Here's how the part is built. I have some questions about the finished solid (model axes, mm). Face numbers are marked on the shaded views. A direction names the side the tool comes from. Give positions to 0.01 mm unless a question says otherwise; leave off trailing zeros. Order: outer loops, then holes, each group sorted by start corner. A loop starts at its lowest first (then second) coordinate and runs counter-clockwise, first axis right, second up. Notation, with made-up numbers: (70.5, 73) - (78.5, 73) arc R31 cw to (78.5, 107) - close; hole circle Ø7 at (25, -8). An arc over 180 degrees is marked (long way). One line per question, with ' | ' between items.
from build123d import *

# Parameters (mm, degrees)
EXTRUDE_1_DEPTH              = 35
CUT_EXTRUDE_2_DEPTH          = 30
SKETCH_2_R                   = 10
SKETCH_2_R_2                 = 15
CUT_EXTRUDE_1_DEPTH          = 1
CUT_EXTRUDE_1_DEPTH_BACK     = 36
EXTRUDE_2_DEPTH              = 5
CUT_EXTRUDE_4_REACH          = 42
SKETCH_11_R                  = 6
EXTRUDE_4_DEPTH              = 35
FILLET_1_R                   = 10
HOLE_WIZARD_M3_1_D           = 2.5
HOLE_WIZARD_M2_1_D           = 1.6
HOLE_WIZARD_M4_1_D           = 3.3
HOLE_WIZARD_M4_2_D           = 4.5
HOLE_WIZARD_M4_2_DEPTH       = 40
HOLE_WIZARD_M4_2_CBORE_D     = 9
HOLE_WIZARD_M4_2_CBORE_DEPTH = 33.1
HOLE_WIZARD_M4_2_TIP         = 1.351936393


with BuildPart() as part:
    # 스케치1 → 보스-돌출1 (new body)
    with BuildSketch(Plane(origin=(0, 0, 0), x_dir=(0, 0, -1), z_dir=(1, 0, 0))):
        with BuildLine():
            Line((-48.263014716, 12.710470067), (81.736985284, 12.710470067))
            ThreePointArc((81.736985284, 12.710470067), (116.736985284, -22.289529933), (81.736985284, -57.289529933))
            Line((81.736985284, -57.289529933), (-48.263014716, -57.289529933))
            ThreePointArc((-48.263014716, -57.289529933), (-83.263014716, -22.289529933), (-48.263014716, 12.710470067))
        make_face()
    extrude(amount=-EXTRUDE_1_DEPTH)

    # 스케치3 → 컷-돌출2 (cut)
    with BuildSketch(Plane.ZY.offset(35)):
        with BuildLine():
            Line((48.263014716, 7.710470067), (-81.736985284, 7.710470067))
            ThreePointArc((-81.736985284, 7.710470067), (-111.736985284, -22.289529933), (-81.736985284, -52.289529933))
            Line((-81.736985284, -52.289529933), (48.263014716, -52.289529933))
            ThreePointArc((48.263014716, -52.289529933), (78.263014716, -22.289529933), (48.263014716, 7.710470067))
        make_face()
    extrude(amount=-CUT_EXTRUDE_2_DEPTH, mode=Mode.SUBTRACT)

    # 스케치2 → 컷-돌출1 (cut, two sides)
    with BuildSketch(Plane(origin=(0, 0, 0), x_dir=(0, 0, -1), z_dir=(1, 0, 0))) as cut_extrude_1_sk:
        with Locations((-23.263014716, -22.302890454)):
            Circle(SKETCH_2_R)
        with Locations((81.736985284, -22.302890454)):
            Circle(SKETCH_2_R_2)
    extrude(amount=CUT_EXTRUDE_1_DEPTH, mode=Mode.SUBTRACT)
    extrude(cut_extrude_1_sk.sketch, amount=-CUT_EXTRUDE_1_DEPTH_BACK, mode=Mode.SUBTRACT)

    # 스케치6 → 보스-돌출2 (add)
    with BuildSketch(Plane.ZY.offset(35)):
        with BuildLine():
            Line((-81.736985284, -54.289529933), (48.263014716, -54.289529933))
            ThreePointArc((48.263014716, -54.289529933), (80.263014716, -22.289529933), (48.263014716, 9.710470067))
            Line((48.263014716, 9.710470067), (-81.736985284, 9.710470067))
            ThreePointArc((-81.736985284, 9.710470067), (-113.736985284, -22.289529933), (-81.736985284, -54.289529933))
        make_face()
        with BuildLine():
            Line((-81.736985284, -52.289529933), (48.263014716, -52.289529933))
            ThreePointArc((48.263014716, -52.289529933), (78.263014716, -22.289529933), (48.263014716, 7.710470067))
            Line((48.263014716, 7.710470067), (-81.736985284, 7.710470067))
            ThreePointArc((-81.736985284, 7.710470067), (-111.736985284, -22.289529933), (-81.736985284, -52.289529933))
        make_face(mode=Mode.SUBTRACT)
    extrude(amount=EXTRUDE_2_DEPTH)

    # 스케치8 → 컷-돌출4 (cut, up to next)
    with BuildSketch(Plane(origin=(0, 0, 0), x_dir=(0, 0, -1), z_dir=(1, 0, 0)), mode=Mode.PRIVATE) as cut_extrude_4_sk1:
        with BuildLine():
            ThreePointArc((76.560604382, -41.608046459), (97.60405209, -10.114301353), (61.736985284, -22.289529933))
            ThreePointArc((61.736985284, -22.289529933), (59.236985284, -24.789529933), (56.736985284, -22.289529933))
            ThreePointArc((56.736985284, -22.289529933), (101.570818791, -7.070494208), (75.266509157, -46.43767559))
            ThreePointArc((75.266509157, -46.43767559), (73.498742204, -43.375813412), (76.560604382, -41.608046459))
        make_face()
    cut_extrude_4_tool1 = extrude(cut_extrude_4_sk1.sketch, amount=-CUT_EXTRUDE_4_REACH, mode=Mode.PRIVATE) & part.part
    add(cut_extrude_4_tool1.solids().sort_by_distance((0, -43.558826, -74.181755))[0], mode=Mode.SUBTRACT)

    # 스케치11 → 보스-돌출4 (add)
    with BuildSketch(Plane.ZY.offset(5)):
        with Locations((-16.736985284, -47.289529933)):
            Circle(SKETCH_11_R)
        with Locations((-16.736985284, 2.710470067)):
            Circle(SKETCH_11_R)
    extrude(amount=EXTRUDE_4_DEPTH)

    # 필렛1
    fillet_1_edges = [part.edges().sort_by_distance(p)[0] for p in [
        (-22.5, -52.289529933, -20.053610075),
        (-22.5, -52.289529933, -13.420360494),
        (-22.5, 7.710470067, -13.420360494),
        (-22.5, 7.710470067, -20.053610075),
    ]]
    fillet(fillet_1_edges, radius=FILLET_1_R)

    # M3 나사 구멍1 (through all)
    with Locations(Plane.ZY.offset(5)):
        with Locations((-62.442692702, -31.965687796), (-68.870568799, -39.626132227)):
            Hole(HOLE_WIZARD_M3_1_D / 2)

    # M2 나사 구멍1 (through all)
    with Locations(Plane.ZY.offset(5)):
        with Locations((-95.142763039, -11.054107284)):
            Hole(HOLE_WIZARD_M2_1_D / 2)

    # M4 나사 구멍1 (through all)
    with Locations(Plane(origin=(0, 0, 0), x_dir=(0, 0, -1), z_dir=(1, 0, 0))):
        with Locations((-53.263014716, -7.302890454), (-53.263014716, -22.302890454), (-53.263014716, -37.302890454), (-33.869616434, -32.909492171), (-33.869616434, -11.696288736), (-12.656412998, -11.696288736), (-12.656412998, -32.909492171)):
            Hole(HOLE_WIZARD_M4_1_D / 2)

    # M4 남비 머리 나사용 카운터보어2
    with Locations(Plane(origin=(0, 0, 0), x_dir=(0, 0, -1), z_dir=(1, 0, 0))):
        with Locations((16.736985284, 2.710470067), (16.736985284, -47.289529933)):
            CounterBoreHole(HOLE_WIZARD_M4_2_D / 2, HOLE_WIZARD_M4_2_CBORE_D / 2, HOLE_WIZARD_M4_2_CBORE_DEPTH, depth=HOLE_WIZARD_M4_2_DEPTH)
            with Locations((0, 0, -(HOLE_WIZARD_M4_2_DEPTH + HOLE_WIZARD_M4_2_TIP / 2))):  # 118° drill point
                Cone(0, HOLE_WIZARD_M4_2_D / 2, HOLE_WIZARD_M4_2_TIP, mode=Mode.SUBTRACT)


solid = part.part
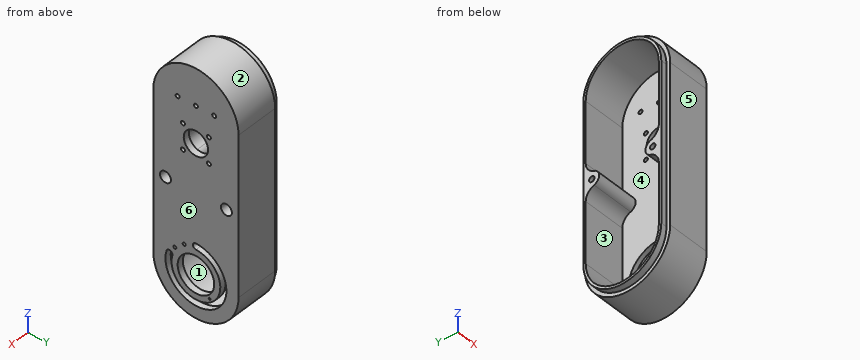
1) On a 3-axis mill with a long thin cutter (end or side, diameter ignored), from which of +Z, -Z, +X, -X, +Y, -Y can I reach the whole of each face in a straight line? I mean the marked faces 1 and 2. Say none if no direction works.
Model answer:
face 1: -X | face 2: +Z, +X, -X
2) I want a section at B-B (z = 28.5). List the corners of the cut face in (x, y) for me.
Model answer:
outline: (-40, -54.29) - (-35, -54.29) - (-35, -57.29) - (0, -57.29) - (0, -30.82) - (-5, -30.82) - (-5, -52.29) - (-40, -52.29) - close; (-40, 7.71) - (-5, 7.71) - (-5, -13.78) - (0, -13.78) - (0, 12.71) - (-35, 12.71) - (-35, 9.71) - (-40, 9.71) - close
3) Thinking about a two-plate mould opening in Y: for the marked faces 3, 4, 5 and 6, which applies, +Y half, -Y half, draft (parallel to the pull), parting line (faces both ways), or undercut?
Model answer:
face 3: undercut | face 4: undercut | face 5: -Y half | face 6: draft
4) I want a section at A-A (x = -11.5). List the corners of the cut face in (y, z) for me.
Model answer:
outline: (-57.29, -81.74) arc R35 ccw to (12.71, -81.74) - (12.71, 48.26) arc R35 ccw to (-57.29, 48.26) - close; hole (-52.29, -81.74) arc R30 ccw to (7.71, -81.74) - (7.71, -31.94) arc R10 ccw to (0.84, -22.44) arc R6 cw to (0.84, -11.04) arc R10 ccw to (7.71, -1.54) - (7.71, 48.26) arc R30 ccw to (-52.29, 48.26) - (-52.29, -1.54) arc R10 ccw to (-45.41, -11.04) arc R6 cw to (-45.41, -22.44) arc R10 ccw to (-52.29, -31.94) - close; hole circle Ø9 at (-47.29, -16.74); hole circle Ø9 at (2.71, -16.74)
5) I want a section at C-C (z = -28.5). List the corners of the cut face in (x, y) for me.
Model answer:
outline: (-40, -54.29) - (-35, -54.29) - (-35, -57.29) - (0, -57.29) - (0, 12.71) - (-35, 12.71) - (-35, 9.71) - (-40, 9.71) - (-40, 7.1) - (-5, 7.1) - (-5, -51.68) - (-40, -51.68) - close
6) Please list where these lines run through material, in increasing order: L1, parallel to Y at x = -19.5, z = 42.5; L2, parallel to Z at x = -30.5, y = -0.5; L3, parallel to Y at x = -2, z = -77.5.
Model answer:
L1: y = -57.29 to -52.29, 7.71 to 12.71 | L2: z = -109.13 to -102.36, -21.81 to -19.89, -13.58 to -11.67, 68.88 to 75.65 | L3: y = -57.29 to -46.93, -41.84 to -36.69, -7.91 to -2.74, 2.35 to 12.71
7) I want a section at D-D (z = -4). List the corners of the cut face in (x, y) for me.
Model answer:
outline: (-40, -54.29) - (-35, -54.29) - (-35, -57.29) - (0, -57.29) - (0, 12.71) - (-35, 12.71) - (-35, 9.71) - (-40, 9.71) - (-40, 7.4) - (-5, 7.4) - (-5, -51.98) - (-40, -51.98) - close
8) I'm going to push flat-ended pins straight in: P1, Ø10, axis at y = 3.5, z = -15.5, coming from the +X side; P2, Ø3, axis at y = -31.97, z = -62.44, coming from the -X side; P3, Ø5, axis at x = -4.5, z = -86.5, coming from the +Y side; P4, Ø4, axis at x = -37.5, z = -27.5, coming from the +Y side. Where does each tip first touch, or does it pass through?
Model answer:
P1: stops at x = 0 | P2: stops at x = -5 | P3: stops at y = 12.64 | P4: stops at y = 9.71
